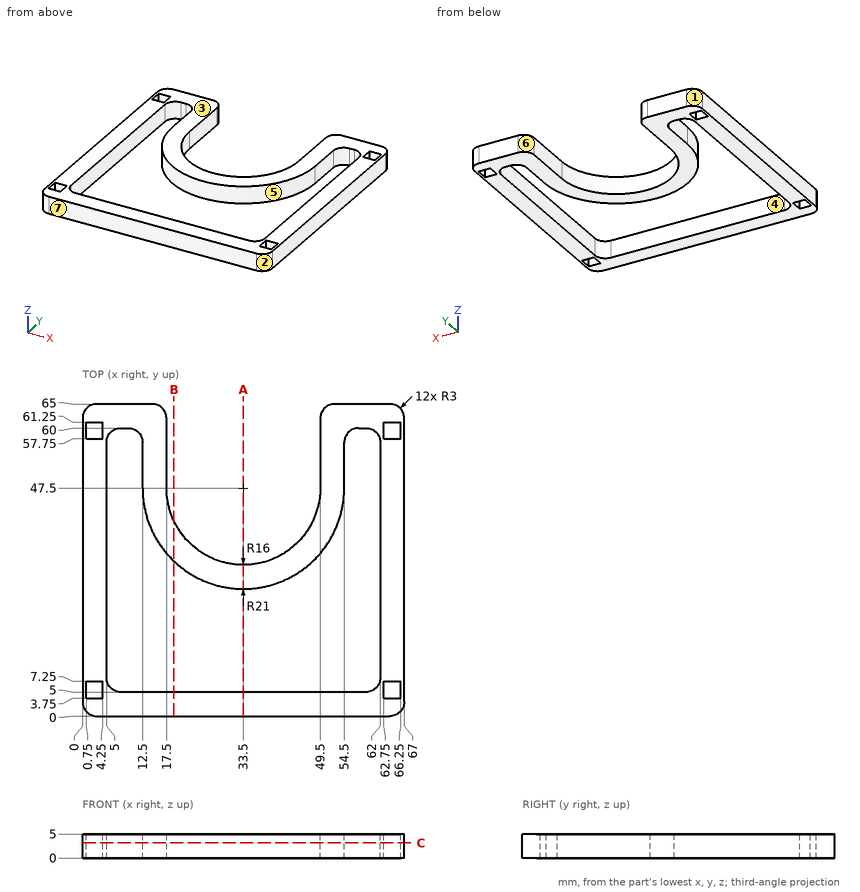
Source: three-view drawing plus pictorial views. Frame: mm from the lowest corner of the part. A direction names the side the tool comes from. Give positions to 0.01 mm unless a question says otherwise; leave off trailing zeros. Write each loop counter-clockwise with the first axis right and the second up, starting at its lowest first coordinate (ties: lowest second). Pieces come first, ordered by that corner, then holes.
(1) Access query for the marked faces 5, 6 and 7. Directions: +Z, -Z, +X, -X, +Y, -Y. A direction counts if a zero-diameter tool reaches every point of the face in a straight line with its end or side. Return the directions, or none.
(2) Ray query, line 1 (X direction, y = 51, z = 2.5); line 2 (Y direction, x = 4, z = 1.05); line 3 (X direction, y = 14, z = 0.75). Return the intervals inside material, ascending.
(3) Cut plane A-A, the plane x = 33.5. Return loops of the section in (y, z), then the cut area to 3 significant figures.
(4) Cut plane B-B, the plane x = 19. Return loops of the section in (y, z), then the cut area to 3 significant figures.
(5) Mould query, pull axis X, two halves, no side actions, for the marked faces 1, 2, 3 and 4. Classes: released by +X, released by -X, zero draft, split by the parting line, or undercut.
(6) Cut plane C-C, the plane z = 3.2. Give the number of separate pieces and of enclosed holes in the cut face, then the cut area to 3 significant figures.
(7) First-contact query: P1, Ø1.5, axis at x = 37.5, z = 3, coming from the +Y side. Flat tip, straight axial feed; report the tip coordinate or a pass-through.
Values follow:
1. face 5: +Z, -Z
1. face 6: +Z, -Z, +Y
1. face 7: +Z, -Z, +X, -X, -Y
2. line 1: x = 0 to 5, 12.5 to 17.5, 49.5 to 54.5, 62 to 67
2. line 2: y = 0 to 3.75, 7.25 to 57.75, 61.25 to 65
2. line 3: x = 0 to 5, 62 to 67
3. outline: (0, 0) - (5, 0) - (5, 5) - (0, 5) - close; (26.5, 0) - (31.5, 0) - (31.5, 5) - (26.5, 5) - close
3. area: 50.0 mm2
4. outline: (0, 0) - (5, 0) - (5, 5) - (0, 5) - close; (32.31, 0) - (40.74, 0) - (40.74, 5) - (32.31, 5) - close
4. area: 67.1 mm2
5. face 1: released by -X
5. face 2: released by +X
5. face 3: zero draft
5. face 4: undercut
6. separate pieces: 1
6. enclosed holes: 5
6. area: 1,430 mm2
7. P1: stops at y = 32.22
